Here's the drawing with two shaded views (mm, measured from the low corner). I have some questions. A direction names the side the tool comes from. Round coordinates to 2 decimals unless told otherwise and drop trailing zeros. Answer as a JSON object with one key per item and string values.
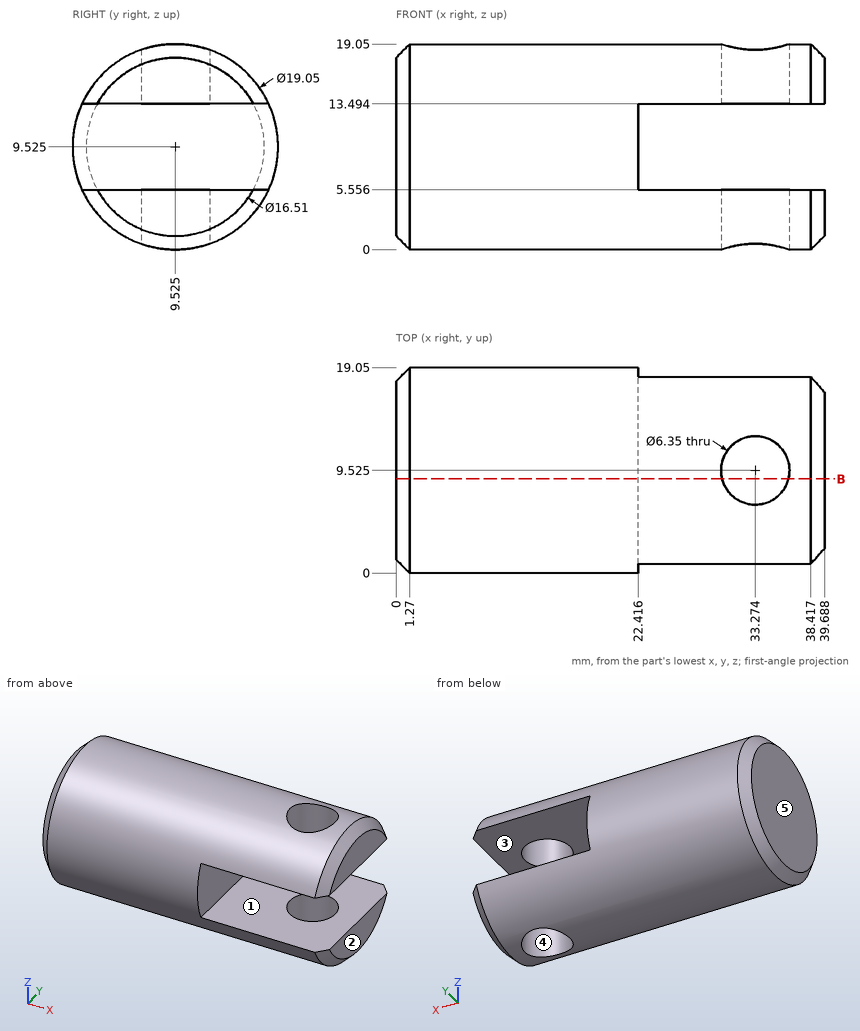
Item 1: If I drill on L1, parallel to X at y = 2.5, z = 9.25 (1 decimal); L2, parallel to Z at x = 30.5, y = 6.25 (1 decimal); L3, parallel to X at y = 10, z = 16 (1 decimal), over which ranges is the centre line in solid material (lowest first)? Write a range as from..to.
Solution:
{"L1": "x = 0..22.4", "L2": "z = 0.6..5.6, 13.5..18.5", "L3": "x = 0..30.1, 36.4..39.7"}
Item 2: I want a section at B-B on y = 8.75. Count the separate pieces of the cut face and the enclosed holes in it, plus the area to 3 significant figures.
Solution:
{"separate pieces": "3", "enclosed holes": "0", "area": "545 mm2"}
Item 3: For the marked faces 1 and 2, which set-ups out of +Z, -Z, +X, -X, +Y, -Y let a thin tool reach every point of the face, with its end or its side?
Solution:
{"face 1": "+X, +Y, -Y", "face 2": "+Z, -Z, +X, +Y, -Y"}
Item 4: For P1, Ø1.5, axis at x = 21.5, y = 7, coming from the -Z side; P2, Ø8, axis at x = 20, z = 2, coming from the +Y side; P3, Ø6, axis at x = 26.5, z = 8.5, coming from the -Y side, each with a flat end and sliding along its axis, tell me the tip position at first contact or that it passes through.
Solution:
{"P1": "stops at z = 0.17", "P2": "stops at y = 18.37", "P3": "stops at y = 0.87"}
Item 5: We'd pull the mould along X, two halves only. Please class the marked faces 3, 4 and 5: +X half, -X half, draft (parallel to the pull), parting line (faces both ways), or undercut.
Solution:
{"face 3": "draft", "face 4": "undercut", "face 5": "-X half"}
